The model under review builds one solid part; all positions refer to its coordinate system, in mm. A direction names the side the tool comes from. Round coordinates to 2 decimals unless told otherwise and drop trailing zeros. Write each loop counter-clockwise with the first axis right and the second up, starting at its lowest first coordinate (ties: lowest second). Pieces come first, ordered by that corner, then holes. Notation, with made-up numbers: (-5, -13) - (38, -13) arc R25 cw to (38, 2) - close; hole circle Ø4 at (-26, -19). An arc over 180 degrees is marked (long way). Use one line per item in the form item = value.
from build123d import *

# Parameters (mm, degrees)
SALIENTE_EXTRUIR1_DEPTH = 12
CROQUIS3_W              = 36
CROQUIS3_H              = 23
CORTAR_EXTRUIR2_DEPTH   = 7
REDONDEO1_R             = 5
CHAFL_N1_SIZE           = 1
CORTAR_EXTRUIR3_DEPTH   = 24
CROQUIS5_R              = 3.5
CORTAR_EXTRUIR4_DEPTH   = 20


with BuildPart() as part:
    # Croquis1 → Saliente-Extruir1 (new body)
    with BuildSketch(Plane.XY):
        with BuildLine():
            Line((216.337020033, 49.627252252), (216.337020033, 26.627252252))
            Line((216.337020033, 26.627252252), (-127.662979967, 26.627252252))
            Line((-127.662979967, 26.627252252), (-127.662979967, 49.627252252))
            Line((-127.662979967, 49.627252252), (74.548659913, 49.627252252))
            ThreePointArc((74.548659913, 49.627252252), (78.30523428, 49.32626093), (76.487020033, 52.627252252))
            Line((76.487020033, 52.627252252), (76.487020033, 66.627252252))
            Line((76.487020033, 66.627252252), (166.337020033, 66.627252252))
            Line((166.337020033, 66.627252252), (166.337020033, 52.627252252))
            ThreePointArc((166.337020033, 52.627252252), (165.940329064, 49.322890173), (169.254470914, 49.627252252))
            Line((169.254470914, 49.627252252), (216.337020033, 49.627252252))
        make_face()
    extrude(amount=SALIENTE_EXTRUIR1_DEPTH)

    # Croquis3 → Cortar-Extruir2 (cut)
    with BuildSketch(Plane(origin=(0, 0, 0), x_dir=(-1, 0, 0), z_dir=(0, 0, -1))):
        with Locations((-51.337020033, 38.127252252)):
            Rectangle(CROQUIS3_W, CROQUIS3_H)
    extrude(amount=-CORTAR_EXTRUIR2_DEPTH, mode=Mode.SUBTRACT)

    # Redondeo1
    redondeo1_edges = [part.edges().sort_by_distance(p)[0] for p in [
        (69.337020033, 38.127252252, 7),
        (33.337020033, 38.127252252, 7),
    ]]
    fillet(redondeo1_edges, radius=REDONDEO1_R)

    # Chaflán1
    chafl_n1_edges = [part.edges().sort_by_distance(p)[0] for p in [
        (33.337020033, 38.127252252, 0),
        (69.337020033, 38.127252252, 0),
    ]]
    chamfer(chafl_n1_edges, length=CHAFL_N1_SIZE)

    # Croquis4 → Cortar-Extruir3 (cut, through all)
    with BuildSketch(Plane(origin=(0, 49.627252252, 0), x_dir=(1, 0, 0), z_dir=(0, 1, 0))):
        with BuildLine():
            Line((-127.662979967, -12), (-127.662979967, -4))
            Line((-127.662979967, -4), (-117.662979967, -4))
            ThreePointArc((-117.662979967, -4), (-112.814866526, -6.70153283), (-111.162979967, -12))
            Line((-111.162979967, -12), (-127.662979967, -12))
        make_face()
    extrude(amount=-CORTAR_EXTRUIR3_DEPTH, mode=Mode.SUBTRACT)

    # Croquis5 → Cortar-Extruir4 (cut)
    with BuildSketch(Plane.XY.offset(14)):
        with Locations((-122.162979967, 37.127252252)):
            Circle(CROQUIS5_R)
    extrude(amount=-CORTAR_EXTRUIR4_DEPTH, mode=Mode.SUBTRACT)


solid = part.part
(1) Add section A-A on z = 9.75. Write out the cut boundary in (x, y).
Geometry results:
outline = (-111.33, 26.63) - (216.34, 26.63) - (216.34, 49.63) - (169.25, 49.63) arc R2.14 cw (long way) to (166.34, 52.63) - (166.34, 66.63) - (76.49, 66.63) - (76.49, 52.63) arc R2.14 cw (long way) to (74.55, 49.63) - (-111.33, 49.63) - close
(2) Insertion check: P1, Ø3, axis at y = 53.5, z = 1.5, coming from the +X side; P2, Ø11, axis at x = -122, y = 36.5, coming from the +Z side; P3, Ø3.5, axis at x = 191, z = 7, coming from the +Y side. Each pin has a flat end and moves straight along its axis. Give the tip position at first contact, or say it passes through.
Geometry results:
P1 = 166.34
P2 = 4.25
P3 = 49.63
(3) Add section B-B on y = 63.5. Write out the cut boundary in (x, z).
Geometry results:
outline = (76.49, 0) - (166.34, 0) - (166.34, 12) - (76.49, 12) - close
(4) To check wall thickness, follow L1, parallel to X at y = 44.5, z = 1.5; L2, parallel to Y at x = -112.5, z = 4.5; L3, parallel to X at y = 62.5, z = 8.5. State the ranges of each line that lie inside material, in increasing order.
Geometry results:
L1 = -127.66 to 33.34, 69.34 to 216.34
L2 = 26.63 to 49.63
L3 = 76.49 to 166.34
(5) Machinability: for faces 1 (the flat face through (55, 42, 12)), 2 (the flat face through (192, 49.627, 6)), 3 (the flat face through (-123, 41, 4)), 4 (the cylindrical face through (-118.825, 38.179, 2.028)), 5 (the flat face through (76.487, 60, 6)), which of the approach directions +Z, -Z, +X, -X, +Y, -Y give a long, thin tool a straight path to every point of the face, cutting with its end or side? Answer none if there is none.
Geometry results:
face_1 = +Z, +X, -X, +Y, -Y
face_2 = +Z, -Z, +X, +Y
face_3 = +Z, -X, +Y, -Y
face_4 = +Z, -Z
face_5 = +Z, -Z, -X, +Y
(6) The part is to be moulded in two halves that separate along X. For faces 6 (the flat face through (128, 47, 0)), 7 (the flat face through (166.337, 60, 6)), 8 (the flat face through (52, 38, 7)), say which applies: +X half, -X half, draft (parallel to the pull), parting line (faces both ways), or undercut.
Geometry results:
face_6 = draft
face_7 = +X half
face_8 = undercut
(7) Add section C-C on x = -2. Write out the cut boundary in (y, z).
Geometry results:
outline = (26.63, 0) - (49.63, 0) - (49.63, 12) - (26.63, 12) - close
